For this review, take the finished solid that the model builds, in its own axes (mm). A direction names the side the tool comes from. Coordinates: 2 decimals unless noted, no trailing zeros. Write each loop counter-clockwise with the first axis right and the second up, starting at its lowest first coordinate (ties: lowest second). Pieces come first, ordered by that corner, then holes. Notation, with made-up numbers: (-11, 89) - (25, 89) arc R32 cw to (25, 116) - close; hole circle Ø2 at (-1.75, 76.25). An arc over 180 degrees is marked (long way). Use one line per item in the form item = value. Start each with the question number.
1) Mouldability with a two-part tool opening along X and no side actions: class faces 6 (the flat face through (136, -5, 41)), 7 (the cylindrical face through (47.245, -9.393, 81.098)), 8 (the flat face through (67, -1, 0)) as pulls with the +X half, pulls with the -X half, needs draft (parallel to the pull), parting line crosses it, or undercut.
2) We need section C-C (y = -7.25). Count the separate pieces of the cut face and the enclosed holes in it, plus the area to 3 significant figures.
3) Insertion check: P1, Ø17.5, axis at x = 14, z = 68, coming from the +Y side; P2, Ø11.5, axis at x = 62.5, z = 26, coming from the -Y side; P3, Ø1.2, axis at y = 2.5, z = 42.5, coming from the +X side. Each pin has a flat end and moves straight along its axis. Give the tip position at first contact, or say it passes through.
4) For L1, parallel to Z at x = 122, y = -7.25; L2, parallel to Z at x = 17.5, y = -3; L3, parallel to X at y = -3.25, z = 19, list the stretches that pass through material, from the lowest coordinate up. Write a range as from..to.
5) We need section A-A (z = 46). Give the boundary of the cut face in (x, y).
6) We need section D-D (x = 53.5). Give the boundary of the cut face in (y, z), plus the area to 3 significant figures.
7) We need section B-B (x = 11). Give the boundary of the cut face in (y, z).
8) Tool access review of faces 1 (the cylindrical face through (19.08, -4.88, 11.89)), 2 (the flat face through (22, 0, 42)), 3 (the cylindrical face through (92.86, -9.41, 81.1)), 4 (the cylindrical face through (49, -6.76, 41.53)), 5 (the cylindrical face through (47.198, -9.393, 0.855)): name each direction out of +Z, -Z, +X, -X, +Y, -Y from which nothing blocks a thin tool from reaching the whole face with its end or side.
```python
from build123d import *

# Parameters (mm, degrees)
F0_W     = 48
F0_H     = 82
F1_DEPTH = 4
F0_R     = 5.5
F2_DEPTH = 9.9
F3_W     = 43.8994949366
F3_H     = 82
F4_DEPTH = 4
F5_F1_R  = 3
F5_F2_R  = 3


with BuildPart() as f1:
    # F0 (on Front) → F1 (new body)
    with BuildSketch(Plane.XZ):
        with Locations((68, 41)):
            Rectangle(F0_W, F0_H)
    extrude(amount=-F1_DEPTH)

    # F0 (on Front) → F2 (join)
    with BuildSketch(Plane.XZ):
        with BuildLine():
            ThreePointArc((0, 14), (4.1005050634, 4.1005050634), (14, 0))
            Line((14, 0), (44, 0))
            Line((44, 0), (44, 82))
            Line((44, 82), (14, 82))
            ThreePointArc((14, 82), (4.1005050634, 77.8994949366), (0, 68))
            Line((0, 68), (0, 14))
        make_face()
        with Locations((14, 14)):
            Circle(F0_R, mode=Mode.SUBTRACT)
        with Locations((14, 68)):
            Circle(F0_R, mode=Mode.SUBTRACT)
        with Locations((68, 41)):
            Rectangle(F0_W, F0_H)
        with BuildLine():
            Line((92, 82), (92, 0))
            Line((92, 0), (122, 0))
            ThreePointArc((122, 0), (131.8994949366, 4.1005050634), (136, 14))
            Line((136, 14), (136, 68))
            ThreePointArc((136, 68), (131.8994949366, 77.8994949366), (122, 82))
            Line((122, 82), (92, 82))
        make_face()
        with Locations((122, 14)):
            Circle(F0_R, mode=Mode.SUBTRACT)
        with Locations((122, 68)):
            Circle(F0_R, mode=Mode.SUBTRACT)
    extrude(amount=F2_DEPTH)

    # F3 (on face) → F4 (cut)
    with BuildSketch(Plane.XZ.offset(9.9)):
        with Locations((70.0502525317, 41)):
            Rectangle(F3_W, F3_H)
    extrude(amount=-F4_DEPTH, mode=Mode.SUBTRACT)

    # F5: fillet of radius 3 on 4 edges, made by hand

    # F5_f1
    f5_f1_edges = [f1.edges().sort_by_distance(p)[0] for p in [
        (48.1005050634, -5.9, 41),
        (92, -5.9, 41),
    ]]
    fillet(f5_f1_edges, radius=F5_F1_R)

    # F5_f2
    f5_f2_edges = [f1.edges().sort_by_distance(p)[0] for p in [
        (70.0502525317, -5.9, 0),
        (70.0502525317, -5.9, 82),
        (91.1213203436, -6.7786796564, 82),
        (48.9791847198, -6.7786796564, 82),
        (48.9791847198, -6.7786796564, 0),
        (91.1213203436, -6.7786796564, 0),
    ]]
    fillet(f5_f2_edges, radius=F5_F2_R)


solid = f1.part
```
Determined:
q1.face_6 = pulls with the +X half
q1.face_7 = undercut
q1.face_8 = needs draft
q2.separate_pieces = 2
q2.enclosed_holes = 4
q2.area = 7,080 mm²
q3.P1 = 0
q3.P2 = -5.9
q3.P3 = 92
q4.L1 = 0..8.5, 19.5..62.5, 73.5..82
q4.L2 = 0..9.76, 18.24..63.76, 72.24..82
q4.L3 = 0..11.71, 16.29..119.71, 124.29..136
q5.outline = (0, -9.9) - (48.1, -9.9) - (48.1, -8.9) arc R3 cw to (51.1, -5.9) - (89, -5.9) arc R3 cw to (92, -8.9) - (92, -9.9) - (136, -9.9) - (136, 0) - (92, 0) - (92, 4) - (44, 4) - (44, 0) - (0, 0) - close
q6.outline = (-5.9, 3) arc R3 ccw to (-2.9, 0) - (4, 0) - (4, 82) - (-2.9, 82) arc R3 ccw to (-5.9, 79) - close
q6.area = 808 mm²
q7.outline = (-9.9, 0.33) - (0, 0.33) - (0, 9.39) - (-9.9, 9.39) - close; (-9.9, 18.61) - (0, 18.61) - (0, 63.39) - (-9.9, 63.39) - close; (-9.9, 72.61) - (0, 72.61) - (0, 81.67) - (-9.9, 81.67) - close
q8.face_1 = +Y, -Y
q8.face_2 = +Z, -Z, -X, +Y
q8.face_3 = +Z, -Y
q8.face_4 = +Z, -Z, -Y
q8.face_5 = -Z, -Y
